```python
from build123d import *

# Parameters (mm, degrees)
SKETCH_W        = 150
SKETCH_H        = 100
PAD_DEPTH       = 5
FILLET_R        = 5
SKETCH001_W     = 10
SKETCH001_H     = 10
PAD001_DEPTH    = 5
FILLET001_R     = 3
FILLET002_R     = 2
SKETCH002_R     = 2.5
POCKET_DEPTH    = 5
SKETCH003_W     = 60
SKETCH003_H     = 50
POCKET001_DEPTH = 5.001
SKETCH004_W     = 14
SKETCH004_H     = 7
POCKET002_DEPTH = 5.001
SKETCH005_W     = 16
SKETCH005_H     = 7
POCKET003_DEPTH = 2
SKETCH006_W     = 16
SKETCH006_H     = 9
POCKET004_DEPTH = 10.001


with BuildPart() as part:
    # Sketch → Pad (new body)
    with BuildSketch(Plane.XY):
        with Locations((75, 50)):
            Rectangle(SKETCH_W, SKETCH_H)
    extrude(amount=PAD_DEPTH)

    # Fillet
    fillet_edges = [part.edges().sort_by_distance(p)[0] for p in [
        (0, 0, 2.5),
        (150, 0, 2.5),
        (150, 100, 2.5),
        (0, 100, 2.5),
    ]]
    fillet(fillet_edges, radius=FILLET_R)

    # Sketch001 → Pad001 (new body)
    with BuildSketch(Plane.XY.offset(5)):
        with Locations((10, 10)):
            Rectangle(SKETCH001_W, SKETCH001_H)
        with Locations((140, 90)):
            Rectangle(SKETCH001_W, SKETCH001_H)
        with Locations((10, 90)):
            Rectangle(SKETCH001_W, SKETCH001_H)
        with Locations((140, 10)):
            Rectangle(SKETCH001_W, SKETCH001_H)
    extrude(amount=PAD001_DEPTH)

    # Fillet001
    fillet001_edges = [part.edges().sort_by_distance(p)[0] for p in [
        (5, 5, 7.5),
        (15, 5, 7.5),
        (5, 15, 7.5),
        (15, 15, 7.5),
        (5, 95, 7.5),
        (15, 95, 7.5),
        (5, 85, 7.5),
        (15, 85, 7.5),
        (135, 5, 7.5),
        (145, 5, 7.5),
        (145, 15, 7.5),
        (135, 85, 7.5),
        (145, 85, 7.5),
        (145, 95, 7.5),
        (135, 95, 7.5),
        (135, 15, 7.5),
    ]]
    fillet(fillet001_edges, radius=FILLET001_R)

    # Fillet002
    fillet002_edges = [part.edges().sort_by_distance(p)[0] for p in [
        (10, 15, 10),
        (140, 15, 10),
        (140, 95, 10),
        (10, 95, 10),
    ]]
    fillet(fillet002_edges, radius=FILLET002_R)

    # Sketch002 → Pocket (cut)
    with BuildSketch(Plane.XY.offset(5)):
        with Locations((56.8, 72.4)):
            Circle(SKETCH002_R)
        with Locations((127, 72.4)):
            Circle(SKETCH002_R)
        with Locations((56.8, 27.6)):
            Circle(SKETCH002_R)
        with Locations((127, 27.6)):
            Circle(SKETCH002_R)
    extrude(amount=-POCKET_DEPTH, mode=Mode.SUBTRACT)

    # Sketch003 → Pocket001 (cut, through all)
    with BuildSketch(Plane.XY.offset(5)):
        with Locations((91.9, 50)):
            Rectangle(SKETCH003_W, SKETCH003_H)
    extrude(amount=-POCKET001_DEPTH, mode=Mode.SUBTRACT)

    # Sketch004 → Pocket002 (cut, through all)
    with BuildSketch(Plane.XY.offset(5)):
        with Locations((27, 71.5)):
            Rectangle(SKETCH004_W, SKETCH004_H)
        with Locations((27, 28.5)):
            Rectangle(SKETCH004_W, SKETCH004_H)
    extrude(amount=-POCKET002_DEPTH, mode=Mode.SUBTRACT)

    # Sketch005 → Pocket003 (cut)
    with BuildSketch(Plane.XY.offset(5)):
        with Locations((27, 71.5)):
            Rectangle(SKETCH005_W, SKETCH005_H)
        with Locations((27, 28.5)):
            Rectangle(SKETCH005_W, SKETCH005_H)
    extrude(amount=-POCKET003_DEPTH, mode=Mode.SUBTRACT)

    # Sketch006 → Pocket004 (cut, through all)
    with BuildSketch(Plane(origin=(0, 0, 0), x_dir=(1, 0, 0), z_dir=(0, 0, -1))):
        with Locations((27, -28.5)):
            Rectangle(SKETCH006_W, SKETCH006_H)
        with Locations((27, -71.5)):
            Rectangle(SKETCH006_W, SKETCH006_H)
    extrude(amount=-POCKET004_DEPTH, mode=Mode.SUBTRACT)


solid = part.part
```
Design review of the part built by this model. Coordinates are the model's own, in mm. A direction names the side the tool comes from. Give positions to 0.01 mm unless a question says otherwise; leave off trailing zeros. Order: outer loops, then holes, each group sorted by start corner. A loop starts at its lowest first (then second) coordinate and runs counter-clockwise, first axis right, second up. Notation, with made-up numbers: (63, -33.75) - (111, -33.75) arc R20 cw to (111, -4.75) - close; hole circle Ø3 at (73, 49). An arc over 180 degrees is marked (long way). Use a Markdown table: item, result. Add a question column.
(1) Mouldability with a two-part tool opening along Y and no side actions: class faces 6 (the face through (135.9, 5.86, 6.52)), 7 (the face through (27, 76, 2)), 8 (the face through (135, 90, 6)), 9 (the face through (144.1, 85.86, 6.52)) as +Y half, -Y half, draft (parallel to the pull), parting line (faces both ways), or undercut.
(2) Add section A-A on y = 27.6. Give the boundary of the cut face in (x, z), then the cut area to 3 significant figures.
(3) Clearance check with flat-ended pins moving along their axes: P1, Ø3, axis at x = 56.8, y = 27.6, coming from the -Z side; P2, Ø1.5, axis at x = 80.5, y = 74.5, coming from the +Z side; P3, Ø2.5, axis at y = 9, z = 7, coming from the -X side; P4, Ø0.9, axis at x = 9.5, z = 6.5, coming from the +Y side. State where each tip first meets the part, or that it passes through.
(4) Add section C-C on z = 1.5. Give the boundary of the cut face in (x, y), then the cut area to 3 significant figures.
(5) Add section D-D on y = 50. Give the boundary of the cut face in (x, z).
(6) Machinability: for faces 1 (the face through (135.9, 14.14, 6.52)), 2 (the face through (10, 5, 6)), 3 (the face through (19, 72, 2)), 4 (the face through (5.9, 85.86, 6.52)), 5 (the face through (144.14, 14.1, 6.52)), which of the approach directions +Z, -Z, +X, -X, +Y, -Y give a long, thin tool a straight path to every point of the face, cutting with its end or side? Answer none if there is none.
(7) Add section B-B on x = 32. Give the boundary of the cut face in (y, z).
(8) Wall thickness on probe 1 along Y at (x, z) = (56.8, 3.3); probe 2 along X at (y, z) = (28, 2.5); probe 3 along X at (y, z) = (66, 3.75): over which ranges is each line inside the solid? List them lowest first. Write a range as [from, to].
Report:
| question | item | result |
|---|---|---|
| 1 | face 6 | -Y half |
| 1 | face 7 | undercut |
| 1 | face 8 | draft |
| 1 | face 9 | undercut |
| 2 | outline | (0, 0) - (19, 0) - (19, 5) - (0, 5) - close; (35, 0) - (54.3, 0) - (54.3, 5) - (35, 5) - close; (59.3, 0) - (61.9, 0) - (61.9, 5) - (59.3, 5) - close; (121.9, 0) - (124.5, 0) - (124.5, 5) - (121.9, 5) - close; (129.5, 0) - (150, 0) - (150, 5) - (129.5, 5) - close |
| 2 | area | 320 mm² |
| 3 | P1 | passes through |
| 3 | P2 | stops at z = 5 |
| 3 | P3 | stops at x = 5 |
| 3 | P4 | stops at y = 95 |
| 4 | outline | (0, 5) arc R5 ccw to (5, 0) - (145, 0) arc R5 ccw to (150, 5) - (150, 95) arc R5 ccw to (145, 100) - (5, 100) arc R5 ccw to (0, 95) - close; hole (19, 24) - (35, 24) - (35, 33) - (19, 33) - close; hole (19, 67) - (35, 67) - (35, 76) - (19, 76) - close; hole circle Ø5 at (56.8, 27.6); hole circle Ø5 at (56.8, 72.4); hole (61.9, 25) - (121.9, 25) - (121.9, 75) - (61.9, 75) - close; hole circle Ø5 at (127, 27.6); hole circle Ø5 at (127, 72.4) |
| 4 | area | 11,600 mm² |
| 5 | outline | (0, 0) - (61.9, 0) - (61.9, 5) - (0, 5) - close; (121.9, 0) - (150, 0) - (150, 5) - (121.9, 5) - close |
| 6 | face 1 | +Z |
| 6 | face 2 | +Z, +X, -X, -Y |
| 6 | face 3 | +Z, -Z |
| 6 | face 4 | +Z, -X |
| 6 | face 5 | +Z, +X |
| 7 | outline | (0, 0) - (24, 0) - (24, 5) - (0, 5) - close; (33, 0) - (67, 0) - (67, 5) - (33, 5) - close; (76, 0) - (100, 0) - (100, 5) - (76, 5) - close |
| 8 | probe 1 | y = [0, 25.1], [30.1, 69.9], [74.9, 100] |
| 8 | probe 2 | x = [0, 19], [35, 54.33], [59.27, 61.9], [121.9, 124.53], [129.47, 150] |
| 8 | probe 3 | x = [0, 61.9], [121.9, 150] |
